Verification items for this drawing (mm, ordinates from the low corner). Give positions to 0.01 mm unless a question says otherwise; leave off trailing zeros. Loops run counter-clockwise (first coordinate to the right, second up) from the corner with the lowest first, then second, coordinate; pieces in that order, holes last. Notation, with made-up numbers: (14, 37) -> (24, 37) arc R21 cw to (24, 53) -> close; hole circle Ø10 at (-30, 70.25). An arc over 180 degrees is marked (long way). Answer in a Markdown table with one row per item. Add a question column.
Q1. Section check B-B on y = 24. Enter the section's corners in (x, z), and give its area (3 significant figures).
Q2. Material ranges on probe 1 along Y at (x, z) = (0.75, 5); probe 2 along Y at (x, z) = (0.5, 37.5); probe 3 along Z at (x, y) = (1.55, 6), recorded low to high.
Q3. Section check C-C on x = 0.45. Enter the section's corners in (y, z).
Q4. Section check A-A on z = 5. Enter the section's corners in (x, y).
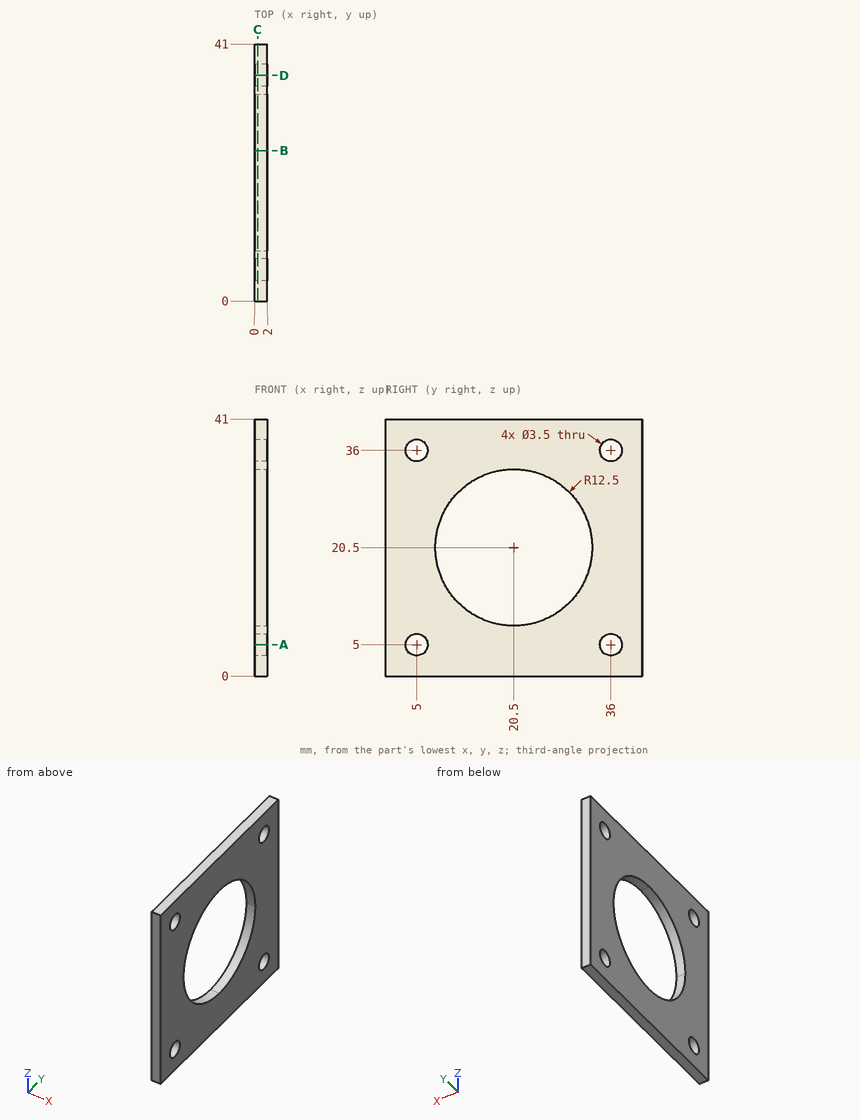
Taken from the geometry:
| question | item | result |
|---|---|---|
| 1 | outline | (0, 0) -> (2, 0) -> (2, 8.5) -> (0, 8.5) -> close; (0, 32.5) -> (2, 32.5) -> (2, 41) -> (0, 41) -> close |
| 1 | area | 34.0 mm² |
| 2 | probe 1 | y = 0 to 3.25, 6.75 to 34.25, 37.75 to 41 |
| 2 | probe 2 | y = 0 to 4.1, 5.9 to 35.1, 36.9 to 41 |
| 2 | probe 3 | z = 0 to 3.56, 6.44 to 34.56, 37.44 to 41 |
| 3 | outline | (0, 0) -> (41, 0) -> (41, 41) -> (0, 41) -> close; hole circle Ø3.5 at (5, 5); hole circle Ø3.5 at (5, 36); hole circle Ø25 at (20.5, 20.5); hole circle Ø3.5 at (36, 5); hole circle Ø3.5 at (36, 36) |
| 4 | outline | (0, 0) -> (2, 0) -> (2, 3.25) -> (0, 3.25) -> close; (0, 6.75) -> (2, 6.75) -> (2, 34.25) -> (0, 34.25) -> close; (0, 37.75) -> (2, 37.75) -> (2, 41) -> (0, 41) -> close |
